Verification items for the finished model (mm, model axes). A direction names the side the tool comes from. Round coordinates to 2 decimals unless told otherwise and drop trailing zeros. Loops run counter-clockwise (first coordinate to the right, second up) from the corner with the lowest first, then second, coordinate; pieces in that order, holes last. Notation, with made-up numbers: M -26.5,55 L 17.5,55 A29 ccw 17.5,80 Z; hole C 33.5,-19.5 d11. An arc over 180 degrees is marked long. Answer as CSV lines item,"result".
```python
from build123d import *

# Parameters (mm, degrees)
F0_R     = 2.5
F1_DEPTH = 3
F2_R     = 1.5
F3_DEPTH = 1
F5_R     = 0.5
F6_DEPTH = 7.501
F7_W     = 2.6
F7_H     = 1
F8_DEPTH = 4.001
F9_R     = 0.2


# Not quite as in the source:
# - a fillet or chamfer that OpenCascade refuses, or shapes differently, is made with other operations: its cross-section is extruded or revolved along the edge and cut away or added


with BuildPart() as f1:
    # F0 (on Top) → F1 (new body)
    with BuildSketch(Plane.XY):
        Circle(F0_R)
    extrude(amount=F1_DEPTH)

    # F2 (on face) → F3 (join)
    with BuildSketch(Plane(origin=(0, 0, 0), x_dir=(1, 0, 0), z_dir=(0, 0, -1))):
        Circle(F2_R)
    extrude(amount=F3_DEPTH)

    # F5 (on offset) → F6 (cut, through all)
    with BuildSketch(Plane.XZ.offset(5)):
        with Locations((0, 1.5)):
            Circle(F5_R)
    extrude(amount=-F6_DEPTH, mode=Mode.SUBTRACT)

    # F7 (on face) → F8 (cut, through all)
    with BuildSketch(Plane.XY.offset(3)):
        Rectangle(F7_W, F7_H)
    extrude(amount=-F8_DEPTH, mode=Mode.SUBTRACT)

    # F9
    f9_edges = [f1.edges().sort_by_distance(p)[0] for p in [
        (-1.3, 0.5, 1),
        (-1.3, -0.5, 1),
        (1.3, -0.5, 1),
        (1.3, 0.5, 1),
    ]]
    fillet(f9_edges, radius=F9_R)

    # F10: chamfer of 0.2 on 3 edges, made by hand

    # F10_s1 → F10_t2 (revolve, cut)
    with BuildSketch(Plane.XZ):
        Polygon((2.3, 3), (2.5, 2.8), (2.5, 3), align=None)
    revolve(axis=Axis((0, 0, 3), (0, 0, 1)), mode=Mode.SUBTRACT)

    # F10_s3 → F10_t4 (revolve, cut)
    with BuildSketch(Plane.XZ):
        Polygon((2.5, 0.2), (2.3, 0), (2.5, 0), align=None)
    revolve(axis=Axis((0, 0, 0), (0, 0, 1)), mode=Mode.SUBTRACT)

    # F10_s5 → F10_t6 (revolve, cut)
    with BuildSketch(Plane.XZ):
        Polygon((1.3, -1), (1.5, -0.8), (1.5, -1), align=None)
    revolve(axis=Axis((0, 0, -1), (0, 0, -1)), mode=Mode.SUBTRACT)


solid = f1.part
```
1) Set-up check for faces 1 (the flat face through (0, 0.5, 0.6)), 2 (the flat face through (0, 1, -1)), 3 (the flat face through (0, -2, 0)): record each of +Z, -Z, +X, -X, +Y, -Y from which the full face is reachable in a straight line by a thin tool's end or side.
Here are the results:
face 1,"+Z, -Z"
face 2,"-Z, +X, -X, +Y, -Y"
face 3,"-Z"
2) Draft check along Y on faces 4 (the cylindrical face through (1.15, -2.22, 1.48)), 5 (the cylindrical face through (0, -2, 2)), 6 (the flat face through (0, -0.5, 0.6)). Enter one of: +Y half, -Y half, draft (parallel to the pull), parting line (faces both ways), or undercut.
Here are the results:
face 4,"parting line"
face 5,"draft"
face 6,"undercut"
3) Section check A-A (y = 0). Record the cut outline in (x, z).
Here are the results:
outline,"M -2.5,0.2 L -2.3,0 L -1.5,0 L -1.5,-0.8 L -1.3,-1 L -1.3,3 L -2.3,3 L -2.5,2.8 Z; M 1.3,-1 L 1.5,-0.8 L 1.5,0 L 2.3,0 L 2.5,0.2 L 2.5,2.8 L 2.3,3 L 1.3,3 Z"
4) Go/stop test with a flat-tipped pin: pin 1 (2 mm diameter, centred on y = -2, z = 0, fed in from +X). Record where the tip stops, or that it passes through.
Here are the results:
pin 1,"stops at x = 2.28"
5) Section check B-B (x = 0). Record the cut outline in (y, z), plus the area to 3 significant figures.
Here are the results:
outline,"M -2.5,0.2 L -2.3,0 L -1.5,0 L -1.5,-0.8 L -1.3,-1 L -0.5,-1 L -0.5,1 L -2.5,1 Z; M -2.5,2 L -0.5,2 L -0.5,3 L -2.3,3 L -2.5,2.8 Z; M 0.5,-1 L 1.3,-1 L 1.5,-0.8 L 1.5,0 L 2.3,0 L 2.5,0.2 L 2.5,1 L 0.5,1 Z; M 0.5,2 L 2.5,2 L 2.5,2.8 L 2.3,3 L 0.5,3 Z"
area,"9.88 mm^2"
6) Material ranges on probe 1 along Z at (x, y) = (0, 1.8); probe 2 along Z at (x, y) = (0, 1.05); probe 3 along X at (y, z) = (2, 1.5), recorded low to high.
Here are the results:
probe 1,"z = 0 to 1, 2 to 3"
probe 2,"z = -1 to 1, 2 to 3"
probe 3,"x = -1.5 to -0.5, 0.5 to 1.5"
7) Section check D-D (z = 1.5). Record the cut outline in (x, y).
Here are the results:
outline,"M -1.3,-0.3 L -1.3,0.3 A0.2 cw -1.1,0.5 L -0.5,0.5 L -0.5,2.45 A2.5 ccw -0.5,-2.45 L -0.5,-0.5 L -1.1,-0.5 A0.2 cw Z; M 0.5,-2.45 A2.5 ccw 0.5,2.45 L 0.5,0.5 L 1.1,0.5 A0.2 cw 1.3,0.3 L 1.3,-0.3 A0.2 cw 1.1,-0.5 L 0.5,-0.5 Z"
8) Section check C-C (z = 0.85). Record the cut outline in (x, y), plus the area to 3 significant figures.
Here are the results:
outline,"C 0,0 d5; hole M -1.3,-0.3 A0.2 ccw -1.1,-0.5 L 1.1,-0.5 A0.2 ccw 1.3,-0.3 L 1.3,0.3 A0.2 ccw 1.1,0.5 L -1.1,0.5 A0.2 ccw -1.3,0.3 Z"
area,"17.1 mm^2"
